Build history of the part. All positions in model axes, mm. A direction names the side the tool comes from. Round coordinates to 2 decimals unless told otherwise and drop trailing zeros. Loops run counter-clockwise (first coordinate to the right, second up) from the corner with the lowest first, then second, coordinate; pieces in that order, holes last. Notation, with made-up numbers: M 40.5,17 L 65.5,17 A24 ccw 65.5,43 Z; hole C 72.5,28.5 d5. An arc over 180 degrees is marked long. One line per item, written item: value.
```python
from build123d import *

# Parameters (mm, degrees)
SKETCH_1_W           = 200
SKETCH_1_H           = 380
EXTRUDE_1_DEPTH      = 10
SKETCH_2_R           = 11
CUT_EXTRUDE_1_DEPTH  = 430.534631898
SKETCH_3_R           = 8
CUT_EXTRUDE_2_DEPTH  = 430.534631898
SKETCH_4_R           = 9.5
CUT_EXTRUDE_3_DEPTH  = 6
CUT_EXTRUDE_START    = -6
SKETCH_5_R           = 9.5
CUT_EXTRUDE_4_DEPTH  = 6
SKETCH_6_R           = 11
CUT_EXTRUDE_5_DEPTH  = 430.534631898
SKETCH_7_R           = 8
CUT_EXTRUDE_6_DEPTH  = 430.534631898
SKETCH_8_R           = 9.5
CUT_EXTRUDE_7_DEPTH  = 6
SKETCH_9_R           = 9.5
CUT_EXTRUDE_8_DEPTH  = 6
SKETCH_10_W          = 40
SKETCH_10_H          = 380
EXTRUDE_3_DEPTH      = 10
CUT_EXTRUDE_9_DEPTH  = 450.55533586
CHAMFER_1_SIZE       = 100
FILLET_1_R           = 30
CUT_EXTRUDE_10_DEPTH = 450.55533586


with BuildPart() as part:
    # 草图1 → 凸台-拉伸1 (new body)
    with BuildSketch(Plane.XY):
        with Locations((100, 190)):
            Rectangle(SKETCH_1_W, SKETCH_1_H)
    extrude(amount=EXTRUDE_1_DEPTH)

    # 草图2 → 切除-拉伸1 (cut, through all)
    with BuildSketch(Plane.XY.offset(10)):
        with Locations((120, 20)):
            Circle(SKETCH_2_R)
        with Locations((145, 63.301270189)):
            Circle(SKETCH_2_R)
    extrude(amount=-CUT_EXTRUDE_1_DEPTH, mode=Mode.SUBTRACT)

    # 草图3 → 切除-拉伸2 (cut, through all)
    with BuildSketch(Plane.XY.offset(10)):
        with Locations((50, 243)):
            Circle(SKETCH_3_R)
    extrude(amount=-CUT_EXTRUDE_2_DEPTH, mode=Mode.SUBTRACT)

    # 草图4 → 切除-拉伸3 (cut)
    with BuildSketch(Plane.XY.offset(10)):
        with Locations((50, 243)):
            Circle(SKETCH_4_R)
    extrude(amount=-CUT_EXTRUDE_3_DEPTH, mode=Mode.SUBTRACT)

    # 草图5 → 切除-拉伸4 (cut)
    with BuildSketch(Plane(origin=(0, 0, 0), x_dir=(-1, 0, 0), z_dir=(0, 0, -1)).offset(CUT_EXTRUDE_START)):
        with Locations(Location((-50, 243, 0), (0, 0, 180))):
            Circle(SKETCH_5_R)
    extrude(amount=CUT_EXTRUDE_4_DEPTH, mode=Mode.SUBTRACT)

    # 草图6 → 切除-拉伸5 (cut, through all)
    with BuildSketch(Plane.XY.offset(10)):
        with Locations((95, 316.698729811)):
            Circle(SKETCH_6_R)
        with Locations((120, 360)):
            Circle(SKETCH_6_R)
    extrude(amount=-CUT_EXTRUDE_5_DEPTH, mode=Mode.SUBTRACT)

    # 草图7 → 切除-拉伸6 (cut, through all)
    with BuildSketch(Plane.XY.offset(10)):
        with Locations((190, 137)):
            Circle(SKETCH_7_R)
    extrude(amount=-CUT_EXTRUDE_6_DEPTH, mode=Mode.SUBTRACT)

    # 草图8 → 切除-拉伸7 (cut)
    with BuildSketch(Plane.XY.offset(10)):
        with Locations((190, 137)):
            Circle(SKETCH_8_R)
    extrude(amount=-CUT_EXTRUDE_7_DEPTH, mode=Mode.SUBTRACT)

    # 草图9 → 切除-拉伸8 (cut)
    with BuildSketch(Plane(origin=(0, 0, 0), x_dir=(-1, 0, 0), z_dir=(0, 0, -1)).offset(CUT_EXTRUDE_START)):
        with Locations(Location((-190, 137, 0), (0, 0, 180))):
            Circle(SKETCH_9_R)
    extrude(amount=CUT_EXTRUDE_8_DEPTH, mode=Mode.SUBTRACT)

    # 草图10 → 凸台-拉伸3 (add)
    with BuildSketch(Plane.XY.offset(10)):
        with Locations((220, 190)):
            Rectangle(SKETCH_10_W, SKETCH_10_H)
    extrude(amount=-EXTRUDE_3_DEPTH)

    # 草图11 → 切除-拉伸9 (cut, through all)
    with BuildSketch(Plane.XY.offset(10)):
        Polygon((240, 185.32943641), (133, 0), (240, 0), align=None)
        Polygon((0, 380), (0, 194.67056359), (107, 380), align=None)
    extrude(amount=-CUT_EXTRUDE_9_DEPTH, mode=Mode.SUBTRACT)

    # 倒角1
    chamfer_1_edges = [part.edges().sort_by_distance(p)[0] for p in [
        (240, 380, 5),
        (0, 0, 5),
    ]]
    chamfer(chamfer_1_edges, length=CHAMFER_1_SIZE)

    # 圆角1
    fillet_1_edges = [part.edges().sort_by_distance(p)[0] for p in [
        (240, 280, 5),
        (140, 380, 5),
        (100, 0, 5),
        (0, 100, 5),
        (240, 185.32943641, 5),
        (133, 0, 5),
        (107, 380, 5),
        (0, 194.67056359, 5),
    ]]
    fillet(fillet_1_edges, radius=FILLET_1_R)

    # 草图12 → 切除-拉伸10 (cut, through all)
    with BuildSketch(Plane.XY.offset(10)):
        with BuildLine():
            Line((28.082053888, 128.486488607), (24.42179985, 132.146742645))
            ThreePointArc((24.42179985, 132.146742645), (21.578419048, 137.912548534), (22.832613624, 144.217810457))
            Line((22.832613624, 144.217810457), (129.975855095, 329.795348372))
            ThreePointArc((129.975855095, 329.795348372), (137.330847211, 334.709796986), (145.707176945, 331.866416184))
            Line((145.707176945, 331.866416184), (149.367430983, 328.206162146))
            ThreePointArc((149.367430983, 328.206162146), (152.210811785, 322.440356256), (150.956617209, 316.135094334))
            Line((150.956617209, 316.135094334), (43.813375738, 130.557556419))
            ThreePointArc((43.813375738, 130.557556419), (36.458383622, 125.643107805), (28.082053888, 128.486488607))
        make_face()
        with BuildLine():
            Line((165.331194154, 294.440009313), (58.187952683, 108.862471397))
            ThreePointArc((58.187952683, 108.862471397), (56.933758108, 102.557209475), (59.777138909, 96.791403586))
            Line((59.777138909, 96.791403586), (63.437392947, 93.131149548))
            ThreePointArc((63.437392947, 93.131149548), (71.813722681, 90.287768746), (79.168714797, 95.20221736))
            Line((79.168714797, 95.20221736), (186.311956268, 280.779755275))
            ThreePointArc((186.311956268, 280.779755275), (187.566150844, 287.085017197), (184.722770042, 292.850823087))
            Line((184.722770042, 292.850823087), (181.062516004, 296.511077125))
            ThreePointArc((181.062516004, 296.511077125), (172.68618627, 299.354457927), (165.331194154, 294.440009313))
        make_face()
        with BuildLine():
            Line((200.686533214, 259.084670253), (93.543291743, 73.507132338))
            ThreePointArc((93.543291743, 73.507132338), (92.289097167, 67.201870416), (95.132477969, 61.436064526))
            Line((95.132477969, 61.436064526), (98.792732007, 57.775810488))
            ThreePointArc((98.792732007, 57.775810488), (107.169061741, 54.932429686), (114.524053856, 59.8468783))
            Line((114.524053856, 59.8468783), (221.667295327, 245.424416216))
            ThreePointArc((221.667295327, 245.424416216), (222.921489903, 251.729678138), (220.078109101, 257.495484027))
            Line((220.078109101, 257.495484027), (216.417855063, 261.155738065))
            ThreePointArc((216.417855063, 261.155738065), (208.041525329, 263.999118867), (200.686533214, 259.084670253))
        make_face()
    extrude(amount=-CUT_EXTRUDE_10_DEPTH, mode=Mode.SUBTRACT)


solid = part.part
```
Item 1: Pull direction X, two halves, no side cores. Call faces 1 (the face through (0, 149, 5)), 2 (the face through (93.568, 327.605, 5.07)), 3 (the face through (47.941, 252.274, 5.07)): pulls with the +X half, pulls with the -X half, needs draft (parallel to the pull), parting line crosses it, or undercut.
Check values:
face 1: pulls with the -X half
face 2: undercut
face 3: undercut
Item 2: Drop flat-ended pins along their axis: P1, Ø17.5, axis at x = 95, y = 316.7, coming from the +Z side; P2, Ø1.5, axis at y = 191.5, z = 7, coming from the -X side; P3, Ø3, axis at x = 168, z = 1.5, coming from the +Y side; P4, Ø6, axis at y = 157, z = 1.5, coming from the +X side. Give the stop position or say it passes through.
Check values:
P1: passes through
P2: stops at x = 0.28
P3: stops at y = 353.5
P4: stops at x = 225.38
Item 3: Wall check: line 1 along Y through (x, z) = (95, 7.75); line 2 along Y through (x, z) = (181.5, 5.75); line 3 along X through (y, z) = (119.5, 4.25). Give the ranges that are in metal, low to high.
Check values:
line 1: y = 5.58 to 61.57, 76.03 to 122.62, 172.62 to 219.22, 269.22 to 305.7, 327.7 to 359.22
line 2: y = 84 to 132.76, 141.24 to 175.85, 225.85 to 272.45, 296.07 to 338.5
line 3: x = 0 to 64.33, 93.2 to 120.1, 148.96 to 201.99
Item 4: Which spindle directions (+Z, -Z, +X, -X, +Y, -Y) get a long thin tool onto all of the face, cutting with end or side? Do faces 4 (the face through (109.13, 375.87, 4.93)), 5 (the face through (152.2, 322.53, 5.07)). Say none if no direction does.
Check values:
face 4: +Z, -Z, -X, +Y
face 5: +Z, -Z
Item 5: Slice it at A-A, the plane y = 20. Give the cut face in (x, z).
Check values:
outline: M 80,0 L 109,0 L 109,10 L 80,10 Z; M 131,0 L 144.55,0 L 144.55,10 L 131,10 Z
Item 6: Slice it at C-C, the plane y = 137. Give the cut face in (x, z), and give its area (3 significant figures).
Check values:
outline: M 0,0 L 21.74,0 L 21.74,10 L 0,10 Z; M 47.53,0 L 74.43,0 L 74.43,10 L 47.53,10 Z; M 103.3,0 L 130.2,0 L 130.2,10 L 103.3,10 Z; M 159.07,0 L 180.5,0 L 180.5,10 L 159.07,10 Z; M 199.5,0 L 212.1,0 L 212.1,10 L 199.5,10 Z
area: 1,100 mm2
Item 7: Slice it at D-D, the plane y = 224.5. Give the cut face in (x, z), and give its area (3 significant figures).
Check values:
outline: M 17.22,0 L 69.18,0 L 69.18,10 L 17.22,10 Z; M 98.05,0 L 124.95,0 L 124.95,10 L 98.05,10 Z; M 153.82,0 L 180.72,0 L 180.72,10 L 153.82,10 Z; M 209.59,0 L 240,0 L 240,10 L 209.59,10 Z
area: 1,360 mm2
Item 8: Slice it at B-B, the plane x = 50. Give the cut face in (y, z).
Check values:
outline: M 50,0 L 141.27,0 L 141.27,10 L 50,10 Z; M 191.27,0 L 233.5,0 L 233.5,10 L 191.27,10 Z; M 252.5,0 L 281.27,0 L 281.27,10 L 252.5,10 Z
